Print and shaded views of the part. All mm, measured from the part's lowest x, y and z. Coordinates: 2 decimals unless noted, no trailing zeros. Order: outer loops, then holes, each group sorted by start corner. A loop starts at its lowest first (then second) coordinate and runs counter-clockwise, first axis right, second up. Notation, with made-up numbers: M 80.25,81.5 L 90.25,81.5 A25 cw 90.25,94.5 Z; hole C 13,-8.5 d7. An arc over 180 degrees is marked long. Return JSON: item names as keys, results as strings.
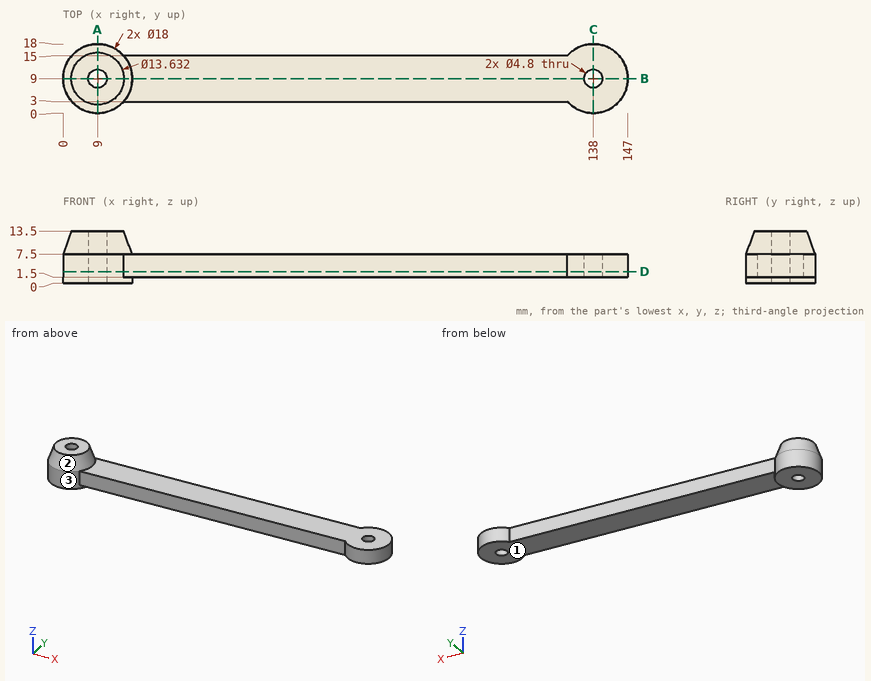
Item 1: Saw through at A-A (x = 9). Write the cut outline in (y, z).
Check result:
{"outline": "M 0,0 L 6.6,0 L 6.6,13.5 L 2.18,13.5 L 0,7.5 Z; M 11.4,0 L 18,0 L 18,7.5 L 15.82,13.5 L 11.4,13.5 Z"}
Item 2: Saw through at B-B (y = 9). Write the cut outline in (x, z).
Check result:
{"outline": "M 0,0 L 6.6,0 L 6.6,13.5 L 2.18,13.5 L 0,7.5 Z; M 11.4,0 L 18,0 L 18,1.5 L 135.6,1.5 L 135.6,7.5 L 18,7.5 L 15.82,13.5 L 11.4,13.5 Z; M 140.4,1.5 L 147,1.5 L 147,7.5 L 140.4,7.5 Z"}
Item 3: Saw through at C-C (x = 138). Write the cut outline in (y, z), and give its area (3 significant figures).
Check result:
{"outline": "M 0,1.5 L 6.6,1.5 L 6.6,7.5 L 0,7.5 Z; M 11.4,1.5 L 18,1.5 L 18,7.5 L 11.4,7.5 Z", "area": "79.2 mm2"}
Item 4: Wall check: line 1 (Y direction, x = 138, z = 3.8); line 2 (X direction, y = 9.5, z = 3.25); line 3 (Z direction, x = 117, y = 12). Give the ranges that are in metal, low to high.
Check result:
{"line 1": "y = 0 to 6.6, 11.4 to 18", "line 2": "x = 0.01 to 6.65, 11.35 to 135.65, 140.35 to 146.99", "line 3": "z = 1.5 to 7.5"}
Item 5: Pull direction X, two halves, no side cores. Call the marked faces 1, 2 and 3: +X half, -X half, draft (parallel to the pull), parting line (faces both ways), or undercut.
Check result:
{"face 1": "draft", "face 2": "parting line", "face 3": "undercut"}
Item 6: Saw through at D-D (z = 3). Write the cut outline in (x, y).
Check result:
{"outline": "M 15.71,3 L 131.29,3 A9 ccw long 131.29,15 L 15.71,15 A9 ccw long Z; hole C 9,9 d4.8; hole C 138,9 d4.8"}
Item 7: Drop flat-ended pins along their axis: pin 1 Ø5 at (x, z) = (62.5, 4.5) entering from -Y; pin 2 Ø3 at (x, z) = (67, 6.5) entering from +Y; pin 3 Ø1.5 at (y, z) = (5, 8.5) entering from -X; pin 4 Ø1.5 at (y, z) = (8.5, 4) entering from -X. Give the stop position or say it passes through.
Check result:
{"pin 1": "stops at y = 3", "pin 2": "stops at y = 15", "pin 3": "stops at x = 0.88", "pin 4": "stops at x = 0"}
